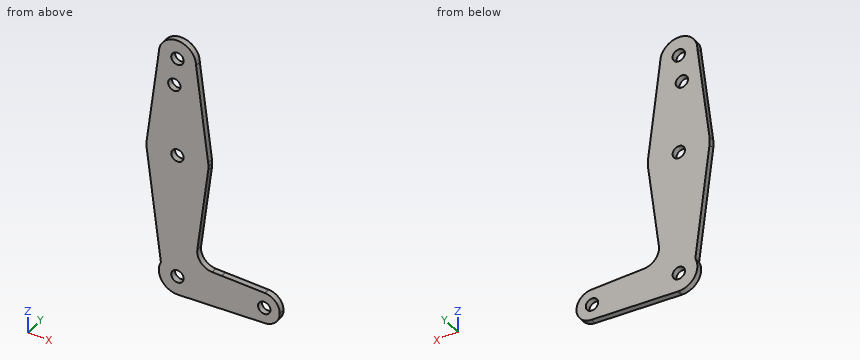
```python
from build123d import *

# Parameters (mm, degrees)
F0_R     = 3.175
F1_DEPTH = 3.048


# Not quite as in the source:
# - ends of sketch curves that miss each other by under 0.0002 mm in the source are joined


with BuildPart() as f1:
    # F0 (on Front) → F1 (new body)
    with BuildSketch(Plane.XZ):
        with BuildLine():
            ThreePointArc((-9.525, 114.3), (0, 104.775), (9.525, 114.3))
            ThreePointArc((9.525, 114.3), (0, 123.825), (-9.525, 114.3))
        make_face()
        with Locations((0, 114.3)):
            Circle(F0_R, mode=Mode.SUBTRACT)
        with BuildLine():
            Line((15.7474569047, 65.5082893304), (9.525, 114.3))
            ThreePointArc((9.525, 114.3), (0, 104.775), (-9.525, 114.3))
            Line((-9.525, 114.3), (-15.7474569047, 65.5082893304))
            ThreePointArc((-15.7474569047, 65.5082893304), (0, 79.375), (15.7474569047, 65.5082893304))
        make_face()
        with Locations((-1.5875, 100.0252)):
            Circle(F0_R, mode=Mode.SUBTRACT)
        with BuildLine():
            ThreePointArc((15.875, 63.5), (15.8430821396, 64.5061676396), (15.7474569047, 65.5082893304))
            ThreePointArc((15.7474569047, 65.5082893304), (0, 79.375), (-15.7474569047, 65.5082893304))
            ThreePointArc((-15.7474569047, 65.5082893304), (-15.875, 63.5), (-15.7474569047, 61.4917106696))
            ThreePointArc((-15.7474569047, 61.4917106696), (0, 47.625), (15.7474569047, 61.4917106696))
            ThreePointArc((15.7474569047, 61.4917106696), (15.8430821396, 62.4938323604), (15.875, 63.5))
        make_face()
        with Locations((0, 63.5)):
            Circle(F0_R, mode=Mode.SUBTRACT)
        with BuildLine():
            ThreePointArc((15.7474569047, 61.4917106696), (0, 47.625), (-15.7474569047, 61.4917106696))
            Line((-15.7474569047, 61.4917106696), (-8.4628069595, 4.371100933))
            ThreePointArc((-8.4628069595, 4.371100933), (2.2491541422, 9.2556431783), (9.525, 0))
            ThreePointArc((9.525, 0), (6.9705567315, -6.4912990883), (0.6773435479, -9.500885786))
            Line((0.6773435479, -9.500885786), (44.7324052746, -7.9324746146))
            ThreePointArc((44.7324052746, -7.9324746146), (36.5125, 0), (44.7324052746, 7.9324746146))
            Line((44.7324052746, 7.9324746146), (22.606619146, 8.7201782014))
            Line((22.606619146, 8.7201782014), (17.7823482037, 8.8932352229))
            ThreePointArc((17.7823482037, 8.8932352229), (12.00790709, 11.6916015121), (10.1808634842, 17.8427750365))
            Line((10.1808634842, 17.8427750365), (10.1810293195, 17.844076245))
            Line((10.1810293195, 17.844076245), (15.7474569047, 61.4917106696))
        make_face()
        with BuildLine():
            ThreePointArc((9.525, 0), (2.2491541422, 9.2556431783), (-8.4628069595, 4.371100933))
            ThreePointArc((-8.4628069595, 4.371100933), (-8.1351202015, -4.9543359097), (0, -9.525))
            Line((0, -9.525), (0.6773435479, -9.500885786))
            ThreePointArc((0.6773435479, -9.500885786), (6.9705567315, -6.4912990883), (9.525, 0))
        make_face()
        Circle(F0_R, mode=Mode.SUBTRACT)
        with BuildLine():
            Line((0.6773435479, -9.500885786), (0, -9.525))
            ThreePointArc((0, -9.525), (0.3388863295, -9.5189695375), (0.6773435479, -9.500885786))
        make_face()
        with BuildLine():
            ThreePointArc((44.7324052746, 7.9324746146), (36.5125, 0), (44.7324052746, -7.9324746146))
            ThreePointArc((44.7324052746, -7.9324746146), (50.1616327839, -5.5119104847), (52.3875, 0))
            ThreePointArc((52.3875, 0), (50.1616327839, 5.5119104847), (44.7324052746, 7.9324746146))
        make_face()
        with Locations((44.45, 0)):
            Circle(F0_R, mode=Mode.SUBTRACT)
    extrude(amount=F1_DEPTH)


solid = f1.part
```
The listing builds one solid part. Answer for the finished solid, in the listing's coordinates (mm). Coordinates: 2 decimals unless noted, no trailing zeros. Write each loop counter-clockwise with the first axis right and the second up, starting at its lowest first coordinate (ties: lowest second). Pieces come first, ordered by that corner, then holes. Notation, with made-up numbers: (61.25, -24) - (95.25, -24) arc R34 ccw to (95.25, 7) - close; hole circle Ø8 at (82, 7). An arc over 180 degrees is marked (long way). Return JSON: item names as keys, results as strings. Group by question number.
1. A cutting plane is placed at B-B, the plane z = 58. Determine the outline of the cut face in (x, y).
2. Straight lines are drawn through the part: L1, parallel to X at y = -2.7, z = 114.5; L2, parallel to Z at x = 44.45, y = -2.05 (3 decimals); L3, parallel to Z at x = -4, y = -2.4. For each, find the intervals that lie inside material, in ascending order.
3. Given pin 1 (1 mm diameter, centred on y = -2.5, z = 61, fed in from +X); pin 2 (1.5 mm diameter, centred on y = -2.5, z = 91.5, fed in from -X); pin 3 (1.5 mm diameter, centred on y = -1.5, z = 66, fed in from -X), each flat-ended and moving along its own axis, determine where each tip first touches the part or whether it passes through.
4. A cutting plane is placed at C-C, the plane x = 34.5. Determine the outline of the cut face in (y, z).
5. A cutting plane is placed at A-A, the plane y = -2.1. Give the number of separate pieces and of enclosed holes in the cut face, plus the area to 3 significant figures.
Ans:
{
 "1": {"outline": "(-15.3, -3.05) - (15.3, -3.05) - (15.3, 0) - (-15.3, 0) - close"},
 "2": {"L1": "-9.52 to -3.17, 3.17 to 9.52", "L2": "-7.943 to -3.175, 3.175 to 7.943", "L3": "-8.64 to 97.96, 102.09 to 122.94"},
 "3": {"pin 1": "x = 15.75", "pin 2": "x = -12.53", "pin 3": "x = -15.78"},
 "4": {"outline": "(-3.05, -8.3) - (0, -8.3) - (0, 8.3) - (-3.05, 8.3) - close"},
 "5": {"separate pieces": "1", "enclosed holes": "5", "area": "3,690 mm²"}
}
